from build123d import *

# Parameters (mm, degrees)
SKETCH1_W           = 270
SKETCH1_H           = 25
BOSS_EXTRUDE1_DEPTH = 10
CUT_EXTRUDE1_REACH  = 273.339
SKETCH2_R           = 3.15
FILLET1_R           = 12.5
SKETCH3_R           = 2.25
CUT_EXTRUDE2_DEPTH  = 272.339271024
CUT_EXTRUDE5_REACH  = 273.339
SKETCH5_W           = 7.3
SKETCH5_H           = 4
SKETCH6_R           = 12.75
CUT_EXTRUDE6_DEPTH  = 4
CUT_EXTRUDE7_REACH  = 273.221
SKETCH7_R           = 1.65
CHAMFER1_SIZE       = 1.5
CHAMFER1_SIZE2      = 1.050311307


with BuildPart() as part:
    # Sketch1 → Boss-Extrude1 (new body)
    with BuildSketch(Plane(origin=(0, 0, 0), x_dir=(1, 0, 0), z_dir=(0, 1, 0))):
        with Locations((135, 12.5)):
            Rectangle(SKETCH1_W, SKETCH1_H)
    extrude(amount=BOSS_EXTRUDE1_DEPTH)

    # Sketch2 → Cut-Extrude1 (cut, up to next)
    with BuildSketch(Plane(origin=(0, 10, 0), x_dir=(1, 0, 0), z_dir=(0, 1, 0)), mode=Mode.PRIVATE) as cut_extrude1_sk1:
        with Locations(Location((12.5, 12.5, 0), (0, 0, 270))):
            Circle(SKETCH2_R)
    cut_extrude1_tool1 = extrude(cut_extrude1_sk1.sketch, amount=-CUT_EXTRUDE1_REACH, mode=Mode.PRIVATE) & part.part
    add(cut_extrude1_tool1.solids().sort_by_distance((12.5, 10, -12.5))[0], mode=Mode.SUBTRACT)

    # Fillet1
    fillet1_edges = [part.edges().sort_by_distance(p)[0] for p in [
        (0, 5, 0),
        (0, 5, -25),
    ]]
    fillet(fillet1_edges, radius=FILLET1_R - 0.0001)  # a hair under: the kernel refuses the full size

    # Sketch3 → Cut-Extrude2 (cut, through all)
    with BuildSketch(Plane(origin=(0, 0, -25), x_dir=(-1, 0, 0), z_dir=(0, 0, -1))):
        with Locations((-264.5, 5)):
            Circle(SKETCH3_R)
        with Locations((-250.5, 5)):
            Circle(SKETCH3_R)
    extrude(amount=-CUT_EXTRUDE2_DEPTH, mode=Mode.SUBTRACT)

    # Sketch5 → Cut-Extrude5 (cut, up to next)
    with BuildSketch(Plane(origin=(0, 10, 0), x_dir=(1, 0, 0), z_dir=(0, 1, 0)), mode=Mode.PRIVATE) as cut_extrude5_sk1:
        with Locations((264.5, 19)):
            Rectangle(SKETCH5_W, SKETCH5_H)
    cut_extrude5_tool1 = extrude(cut_extrude5_sk1.sketch, amount=-CUT_EXTRUDE5_REACH, mode=Mode.PRIVATE) & part.part
    # Sketch5 → Cut-Extrude5 (cut, up to next)
    with BuildSketch(Plane(origin=(0, 10, 0), x_dir=(1, 0, 0), z_dir=(0, 1, 0)), mode=Mode.PRIVATE) as cut_extrude5_sk2:
        with Locations((264.5, 6)):
            Rectangle(SKETCH5_W, SKETCH5_H)
    cut_extrude5_tool2 = extrude(cut_extrude5_sk2.sketch, amount=-CUT_EXTRUDE5_REACH, mode=Mode.PRIVATE) & part.part
    # Sketch5 → Cut-Extrude5 (cut, up to next)
    with BuildSketch(Plane(origin=(0, 10, 0), x_dir=(1, 0, 0), z_dir=(0, 1, 0)), mode=Mode.PRIVATE) as cut_extrude5_sk3:
        with Locations((250.5, 19)):
            Rectangle(SKETCH5_W, SKETCH5_H)
    cut_extrude5_tool3 = extrude(cut_extrude5_sk3.sketch, amount=-CUT_EXTRUDE5_REACH, mode=Mode.PRIVATE) & part.part
    # Sketch5 → Cut-Extrude5 (cut, up to next)
    with BuildSketch(Plane(origin=(0, 10, 0), x_dir=(1, 0, 0), z_dir=(0, 1, 0)), mode=Mode.PRIVATE) as cut_extrude5_sk4:
        with Locations((250.5, 6)):
            Rectangle(SKETCH5_W, SKETCH5_H)
    cut_extrude5_tool4 = extrude(cut_extrude5_sk4.sketch, amount=-CUT_EXTRUDE5_REACH, mode=Mode.PRIVATE) & part.part
    add(cut_extrude5_tool1.solids().sort_by_distance((264.5, 10, -19))[0], mode=Mode.SUBTRACT)
    add(cut_extrude5_tool2.solids().sort_by_distance((264.5, 10, -6))[0], mode=Mode.SUBTRACT)
    add(cut_extrude5_tool3.solids().sort_by_distance((250.5, 10, -19))[0], mode=Mode.SUBTRACT)
    add(cut_extrude5_tool4.solids().sort_by_distance((250.5, 10, -6))[0], mode=Mode.SUBTRACT)

    # Sketch6 → Cut-Extrude6 (cut)
    with BuildSketch(Plane.XZ):
        with Locations((12.5, -12.5)):
            Circle(SKETCH6_R)
    extrude(amount=-CUT_EXTRUDE6_DEPTH, mode=Mode.SUBTRACT)

    # Sketch7 → Cut-Extrude7 (cut, up to next)
    with BuildSketch(Plane.XZ.offset(-4), mode=Mode.PRIVATE) as cut_extrude7_sk1:
        with Locations(Location((12.5, -20.5, 0), (0, 0, 270))):
            Circle(SKETCH7_R)
    cut_extrude7_tool1 = extrude(cut_extrude7_sk1.sketch, amount=-CUT_EXTRUDE7_REACH, mode=Mode.PRIVATE) & part.part
    # Sketch7 → Cut-Extrude7 (cut, up to next)
    with BuildSketch(Plane.XZ.offset(-4), mode=Mode.PRIVATE) as cut_extrude7_sk2:
        with Locations(Location((5.57179677, -8.5, 0), (0, 0, 270))):
            Circle(SKETCH7_R)
    cut_extrude7_tool2 = extrude(cut_extrude7_sk2.sketch, amount=-CUT_EXTRUDE7_REACH, mode=Mode.PRIVATE) & part.part
    # Sketch7 → Cut-Extrude7 (cut, up to next)
    with BuildSketch(Plane.XZ.offset(-4), mode=Mode.PRIVATE) as cut_extrude7_sk3:
        with Locations(Location((19.42820323, -8.5, 0), (0, 0, 270))):
            Circle(SKETCH7_R)
    cut_extrude7_tool3 = extrude(cut_extrude7_sk3.sketch, amount=-CUT_EXTRUDE7_REACH, mode=Mode.PRIVATE) & part.part
    add(cut_extrude7_tool1.solids().sort_by_distance((12.5, 4, -20.5))[0], mode=Mode.SUBTRACT)
    add(cut_extrude7_tool2.solids().sort_by_distance((5.571797, 4, -8.5))[0], mode=Mode.SUBTRACT)
    add(cut_extrude7_tool3.solids().sort_by_distance((19.428203, 4, -8.5))[0], mode=Mode.SUBTRACT)

    # Chamfer1
    chamfer1_edges = [part.edges().sort_by_distance(p)[0] for p in [
        (12.5, 10, -18.85),
        (5.57179677, 10, -6.85),
        (19.42820323, 10, -6.85),
    ]]
    chamfer1_side = [part.faces().sort_by_distance(p)[0] for p in [
        (135.233508086, 10, -12.5),
    ]]
    chamfer(chamfer1_edges, length=CHAMFER1_SIZE, length2=CHAMFER1_SIZE2, reference=chamfer1_side[0])


solid = part.part
Verification items for the finished model (mm, model axes). A direction names the side the tool comes from. Give positions to 0.01 mm unless a question says otherwise; leave off trailing zeros. Order: outer loops, then holes, each group sorted by start corner. A loop starts at its lowest first (then second) coordinate and runs counter-clockwise, first axis right, second up. Notation, with made-up numbers: M 72,-37 L 102,-37 A27 cw 102,-19 Z; hole C 54.5,66.25 d11. An arc over 180 degrees is marked long. Answer as a JSON object with one key per item and string values. Group by question number.
1) Scan lines: line 1 along Z through (x, y) = (252, 1); line 2 along X through (y, z) = (8, -12.5); line 3 along X through (y, z) = (3, -10.25). Record each from-to range of solid material in increasing order. Write a range as [from, to].
2) Mould release check, pull along Z, two halves, no side actions. Record for faces 4 (the face through (266.748, 5.099, -2.028)), 5 (the face through (3.564, 7.042, -21.241)), 6 (the face through (12.638, 7.042, -15.647)): released by +Z, released by -Z, zero draft, split by the parting line, or undercut.
3) Access from +Z, -Z, +X, -X, +Y, -Y to the whole of each face (thin tool, end or side, straight path). Record for faces 1 (the face through (25.248, 1.972, -12.745)), 2 (the face through (266.748, 5.099, -12.563)), 3 (the face through (251.3, 7.3, -4)).
4) Cross-section at A-A (x = 250.5). Enter the section's corners in (y, z).
5) Depth check by flat-ended pin: pin 1 Ø4 at (y, z) = (3, -6.5) entering from -X. Enter the tip coordinate at first touch or a pass-through.
Result sheet:
{
 "1": {"line 1": "z = [-25, -21], [-17, -8], [-4, 0]", "line 2": "x = [0, 9.35], [15.65, 270]", "line 3": "x = [25.05, 249.47], [251.53, 263.47], [265.53, 270]"},
 "2": {"face 4": "zero draft", "face 5": "released by -Z", "face 6": "undercut"},
 "3": {"face 1": "-X, -Y", "face 2": "+Z, -Z", "face 3": "+Y, -Y"},
 "4": {"outline": "M 0,-25 L 2.75,-25 L 2.75,-21 L 0,-21 Z; M 0,-17 L 2.75,-17 L 2.75,-8 L 0,-8 Z; M 0,-4 L 2.75,-4 L 2.75,0 L 0,0 Z; M 7.25,-25 L 10,-25 L 10,-21 L 7.25,-21 Z; M 7.25,-17 L 10,-17 L 10,-8 L 7.25,-8 Z; M 7.25,-4 L 10,-4 L 10,0 L 7.25,0 Z"},
 "5": {"pin 1": "stops at x = 0.75"}
}
